The model under review builds one solid part; all positions refer to its coordinate system, in mm. Round coordinates to 2 decimals unless told otherwise and drop trailing zeros. Order: outer loops, then holes, each group sorted by start corner. A loop starts at its lowest first (then second) coordinate and runs counter-clockwise, first axis right, second up.
```python
from build123d import *

# Parameters (mm, degrees)
SKETCH_1_R      = 20
SKETCH_1_R_2    = 2
SKETCH_1_R_3    = 1.4
SKETCH_1_R_4    = 1.5
SKETCH_1_R_5    = 4
EXTRUDE_1_DEPTH = 4


with BuildPart() as part:
    # 草图1 → 凸台-拉伸1 (new body)
    with BuildSketch(Plane.XY):
        Circle(SKETCH_1_R)
        Circle(SKETCH_1_R_2, mode=Mode.SUBTRACT)
        with Locations((6.5, 0)):
            Circle(SKETCH_1_R_3, mode=Mode.SUBTRACT)
        with Locations((0, -15.5)):
            Circle(SKETCH_1_R_4, mode=Mode.SUBTRACT)
        with Locations((-15.5, 0)):
            Circle(SKETCH_1_R_4, mode=Mode.SUBTRACT)
        with Locations((0, 15.5)):
            Circle(SKETCH_1_R_4, mode=Mode.SUBTRACT)
        with Locations((15.5, 0)):
            Circle(SKETCH_1_R_4, mode=Mode.SUBTRACT)
        with Locations(Location((-6.5, 0, 0), (0, 0, 180))):
            Circle(SKETCH_1_R_3, mode=Mode.SUBTRACT)
        with Locations((-7.75, 7.75)):
            Circle(SKETCH_1_R_5, mode=Mode.SUBTRACT)
        with Locations((7.75, 7.75)):
            Circle(SKETCH_1_R_5, mode=Mode.SUBTRACT)
        with Locations((7.75, -7.75)):
            Circle(SKETCH_1_R_5, mode=Mode.SUBTRACT)
        with Locations((-7.75, -7.75)):
            Circle(SKETCH_1_R_5, mode=Mode.SUBTRACT)
    extrude(amount=EXTRUDE_1_DEPTH)


solid = part.part
```
(1) Consider section C-C (x = 0). Write out the cut boundary in (y, z).
Data:
outline: (-20, 0) - (-17, 0) - (-17, 4) - (-20, 4) - close; (-14, 0) - (-2, 0) - (-2, 4) - (-14, 4) - close; (2, 0) - (14, 0) - (14, 4) - (2, 4) - close; (17, 0) - (20, 0) - (20, 4) - (17, 4) - close
(2) Insertion check: pin 1 (6.5 mm diameter, centred on x = 7.75, y = 7.75, fed in from +Z); pin 2 (1.5 mm diameter, centred on x = -4.5, z = 3.5, fed in from +Y); pin 3 (1.5 mm diameter, centred on x = -10.5, z = 3, fed in from -Y); pin 4 (1 mm diameter, centred on y = 6, z = 1.5, fed in from -X). Each pin has a flat end and moves straight along its axis. Give the tip position at first contact, or say it passes through.
Data:
pin 1: passes through
pin 2: stops at y = 19.65
pin 3: stops at y = -17.46
pin 4: stops at x = -19.23
(3) Draft analysis for pull direction X (two halves, no side actions). For faces 1 (the cylindrical face through (3.754, -7.574, 1.972)), 2 (the cylindrical face through (-7.835, -0.421, 1.972)), 3 (the flat face through (0, -4, 4)), 4 (the cylindrical face through (-4.336, -19.524, 1.972)), state which applies: pulls with the +X half, pulls with the -X half, needs draft (parallel to the pull), parting line crosses it, or undercut.
Data:
face 1: undercut
face 2: undercut
face 3: needs draft
face 4: parting line crosses it
(4) Consider section D-D (y = -15.5). Write out the cut boundary in (x, z).
Data:
outline: (-12.64, 0) - (-1.5, 0) - (-1.5, 4) - (-12.64, 4) - close; (1.5, 0) - (12.64, 0) - (12.64, 4) - (1.5, 4) - close
(5) Consider section B-B (z = 0.8). State how many separate pieces and enclosed holes the cut face has, and give its area (3 significant figures).
Data:
separate pieces: 1
enclosed holes: 11
area: 1,000 mm2
(6) Consider section A-A (y = 0). Write out the cut boundary in (x, z), and give its area (3 significant figures).
Data:
outline: (-20, 0) - (-17, 0) - (-17, 4) - (-20, 4) - close; (-14, 0) - (-7.9, 0) - (-7.9, 4) - (-14, 4) - close; (-5.1, 0) - (-2, 0) - (-2, 4) - (-5.1, 4) - close; (2, 0) - (5.1, 0) - (5.1, 4) - (2, 4) - close; (7.9, 0) - (14, 0) - (14, 4) - (7.9, 4) - close; (17, 0) - (20, 0) - (20, 4) - (17, 4) - close
area: 97.6 mm2
(7) To check wall thickness, follow probe 1 along X at (y, z) = (-5.5, 2.2); probe 2 along Y at (x, z) = (7.75, 1.75); probe 3 along X at (y, z) = (7.5, 1.15). State the ranges of each line that lie inside material, in increasing order.
Data:
probe 1: x = -19.23 to -11.06, -4.44 to 4.44, 11.06 to 19.23
probe 2: y = -18.44 to -11.75, -3.75 to -0.63, 0.63 to 3.75, 11.75 to 18.44
probe 3: x = -18.54 to -11.74, -3.76 to 3.76, 11.74 to 18.54
